For this review, take the finished solid that the model builds, in its own axes (mm). Face numbers are marked on the shaded views. A direction names the side the tool comes from. Coordinates: 2 decimals unless noted, no trailing zeros. Loops run counter-clockwise (first coordinate to the right, second up) from the corner with the lowest first, then second, coordinate; pieces in that order, holes last. Notation, with made-up numbers: M -15.75,38.5 L 18.25,38.5 A23 cw 18.25,58.5 Z; hole C 68.5,60.5 d11. An arc over 180 degrees is marked long. Use one line per item in the form item = value.
```python
from build123d import *

# Parameters (mm, degrees)
SKETCH1_R                      = 12.5
BOSS_EXTRUDE1_DEPTH            = 17.6
SKETCH2_R                      = 6.875
CUT_EXTRUDE1_DEPTH             = 50.8
SKETCH3_R                      = 8
CUT_EXTRUDE3_DEPTH             = 15.6
CUT_EXTRUDE4_DEPTH             = 18.6
BOSS_EXTRUDE2_DEPTH            = 17.6
FILLET1_R                      = 4
SKETCH6_W                      = 25
SKETCH6_H                      = 20.775
BOSS_EXTRUDE3_DEPTH            = 20
M4X0_7_TAPPED_HOLE2_AT_2_COUNT = 2
M4X0_7_TAPPED_HOLE2_AT_2_PITCH = 12.206555616
M4X0_7_TAPPED_HOLE1_D          = 3.3
M4X0_7_TAPPED_HOLE1_DEPTH      = 7
M4X0_7_TAPPED_HOLE1_TIP        = 0.991420021
FILLET4_R                      = 1
FILLET6_R                      = 1
FILLET7_R                      = 2
CUT_EXTRUDE6_DEPTH             = 15.6
FILLET8_R                      = 5
BOSS_EXTRUDE4_DEPTH            = 17.6
FILLET11_R                     = 1


with BuildPart() as part:
    # Sketch1 → Boss-Extrude1 (new body)
    with BuildSketch(Plane(origin=(0, 0, 0), x_dir=(1, 0, 0), z_dir=(0, 1, 0))):
        Circle(SKETCH1_R)
    extrude(amount=BOSS_EXTRUDE1_DEPTH)

    # Sketch2 → Cut-Extrude1 (cut)
    with BuildSketch(Plane(origin=(0, 17.6, 0), x_dir=(1, 0, 0), z_dir=(0, 1, 0))):
        Circle(SKETCH2_R)
    extrude(amount=-CUT_EXTRUDE1_DEPTH, mode=Mode.SUBTRACT)

    # Sketch3 → Cut-Extrude3 (cut)
    with BuildSketch(Plane(origin=(0, 17.6, 0), x_dir=(1, 0, 0), z_dir=(0, 1, 0))):
        Circle(SKETCH3_R)
    extrude(amount=-CUT_EXTRUDE3_DEPTH, mode=Mode.SUBTRACT)

    # Sketch4 → Cut-Extrude4 (cut, through all)
    with BuildSketch(Plane(origin=(0, 17.6, 0), x_dir=(1, 0, 0), z_dir=(0, 1, 0))):
        with BuildLine():
            ThreePointArc((-2.736161147, 7.517540966), (2.405646396, 7.629735606), (6.553216354, 4.588611491))
            Line((6.553216354, 4.588611491), (10.239400554, 7.169705454))
            ThreePointArc((10.239400554, 7.169705454), (3.758822494, 11.921461884), (-4.275251792, 11.74615776))
            Line((-4.275251792, 11.74615776), (-2.736161147, 7.517540966))
        make_face()
    extrude(amount=-CUT_EXTRUDE4_DEPTH, mode=Mode.SUBTRACT)

    # Sketch5 → Boss-Extrude2 (add, through all)
    with BuildSketch(Plane(origin=(0, 17.6, 0), x_dir=(1, 0, 0), z_dir=(0, 1, 0))):
        with BuildLine():
            Line((8.100371818, -9.520187835), (32.472052675, 11.216764019))
            Line((32.472052675, 11.216764019), (23.399636239, 21.879374394))
            Line((23.399636239, 21.879374394), (10.717665156, 11.088759446))
            Line((10.717665156, 11.088759446), (10.239400554, 7.169705454))
            ThreePointArc((10.239400554, 7.169705454), (12.398586499, -1.589041484), (8.100371818, -9.520187835))
        make_face()
    extrude(amount=-BOSS_EXTRUDE2_DEPTH)

    # Fillet1
    fillet1_edges = [part.edges().sort_by_distance(p)[0] for p in [
        (-2.736161147, 9.8, -7.517540966),
    ]]
    fillet(fillet1_edges, radius=FILLET1_R)

    # Sketch6 → Boss-Extrude3 (add)
    with BuildSketch(Plane(origin=(24.371680857, 0, -20.736951854), x_dir=(-0.648029745, 0, -0.761615027), z_dir=(0.761615027, 0, -0.648029745))):
        with Locations((0, 10.3875)):
            Rectangle(SKETCH6_W, SKETCH6_H)
    extrude(amount=BOSS_EXTRUDE3_DEPTH)

    # Sketch9 → M4x0.7 Tapped Hole2 (revolve, cut)
    with BuildSketch(Plane(origin=(25.410689361, 15.3875, -38.033496634), x_dir=(-0.761615027, 0, 0.648029745), z_dir=(0, 1, 0))):
        Polygon((0, 0), (0, 7.991420021), (1.65, 7), (1.65, 0), align=None)
    m4x0_7_tapped_hole2 = revolve(axis=Axis((21.295700477, 15.3875, -42.869752054), (0.648029745, 0, 0.761615027)), mode=Mode.SUBTRACT)

    # M4x0.7 Tapped Hole2 at 2: M4x0.7 Tapped Hole2 ×2
    with Locations(*[Vector(-0.436757539, -0.819231921, 0.371620657) * (i * M4X0_7_TAPPED_HOLE2_AT_2_PITCH) for i in range(1, M4X0_7_TAPPED_HOLE2_AT_2_COUNT)]):
        add(m4x0_7_tapped_hole2, mode=Mode.SUBTRACT)

    # Mirror1: M4x0.7 Tapped Hole2 across plane
    add(m4x0_7_tapped_hole2.mirror(Plane(origin=(0, 0, 0), x_dir=(-0.761615027, 0, 0.648029745), z_dir=(-0.648029745, 0, -0.761615027))), mode=Mode.SUBTRACT)

    # Mirror1 copy 1 sketch → Mirror1 copy 1 (revolve, cut)
    with BuildSketch(Plane(origin=(36.280127809, 5.3875, -14.456912746), x_dir=(-0.761615027, 0, 0.648029745), z_dir=(0, 1, 0))):
        Polygon((0, 0), (0, -7.991420021), (1.65, -7), (1.65, 0), align=None)
    revolve(axis=Axis((40.395116693, 5.3875, -9.620657326), (0.648029745, 0, 0.761615027)), mode=Mode.SUBTRACT)

    # M4x0.7 Tapped Hole1
    with Locations(Plane(origin=(0, 17.6, 0), x_dir=(1, 0, 0), z_dir=(0, 1, 0))):
        with Locations((20.785019884, 12.607162838), (15.760988598, 3.080405276)):
            Hole(M4X0_7_TAPPED_HOLE1_D / 2, depth=M4X0_7_TAPPED_HOLE1_DEPTH)
            with Locations((0, 0, -(M4X0_7_TAPPED_HOLE1_DEPTH + M4X0_7_TAPPED_HOLE1_TIP / 2))):  # 118° drill point
                Cone(0, M4X0_7_TAPPED_HOLE1_D / 2, M4X0_7_TAPPED_HOLE1_TIP, mode=Mode.SUBTRACT)

    # Fillet4
    fillet4_edges = [part.edges().sort_by_distance(p)[0] for p in [
        (27.935844457, 17.6, -16.548069207),
    ]]
    fillet(fillet4_edges, radius=FILLET4_R)

    # Fillet6
    fillet6_edges = [part.edges().sort_by_distance(p)[0] for p in [
        (-2.736161147, 1, -7.517540966),
        (6.553216354, 1, -4.588611491),
    ]]
    fillet(fillet6_edges, radius=FILLET6_R)

    # Fillet7
    fillet7_edges = [part.edges().sort_by_distance(p)[0] for p in [
        (23.399636239, 8.8, -21.879374394),
    ]]
    fillet(fillet7_edges, radius=FILLET7_R)

    # Sketch13 → Cut-Extrude6 (cut)
    with BuildSketch(Plane(origin=(0, 17.6, 0), x_dir=(1, 0, 0), z_dir=(0, 1, 0))):
        Polygon((7.237831979, 3.407900857), (11.336580589, 16.160351586), (5.142300877, 6.128355545), (6.34884573, 4.867459081), align=None)
    extrude(amount=-CUT_EXTRUDE6_DEPTH, mode=Mode.SUBTRACT)

    # Fillet8
    fillet8_edges = [part.edges().sort_by_distance(p)[0] for p in [
        (7.237831979, 9.8, -3.407900857),
    ]]
    fillet(fillet8_edges, radius=FILLET8_R)

    # Sketch14 → Boss-Extrude4 (add)
    with BuildSketch(Plane(origin=(0, 17.6, 0), x_dir=(1, 0, 0), z_dir=(0, 1, 0))):
        Polygon((7.926350274, 5.550090213), (9.325919645, 9.904575236), (10.717665156, 11.088759446), (10.239400554, 7.169705454), align=None)
    extrude(amount=-BOSS_EXTRUDE4_DEPTH)

    # Fillet11
    fillet11_edges = [part.edges().sort_by_distance(p)[0] for p in [
        (9.325919645, 8.8, -9.904575236),
    ]]
    fillet(fillet11_edges, radius=FILLET11_R)


solid = part.part
```
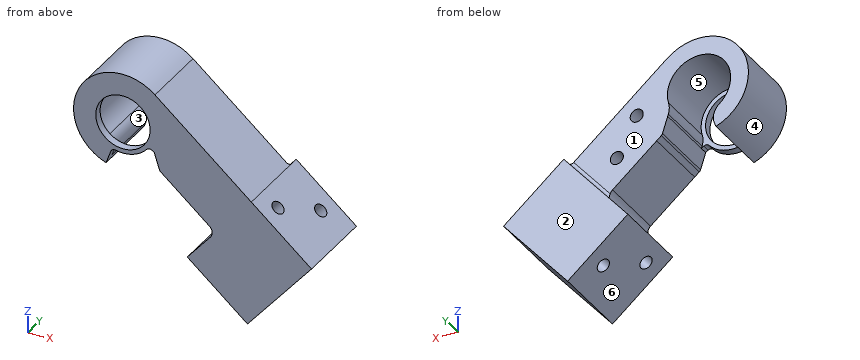
1. Consider section D-D on y = 19.75. Write out the cut boundary in (x, z).
Computed values:
outline = M 16.27,-30.26 L 31.5,-43.22 L 47.7,-24.18 L 32.47,-11.22 Z
2. Consider section B-B on y = 12.5. Write out the cut boundary in (x, z).
Computed values:
outline = M -5.09,-6.18 A8 cw long 7.7,-2.15 A5 ccw 7.76,-5.03 L 9.24,-9.63 A1 ccw 9.54,-10.09 L 21.88,-20.58 A2 cw 22.1,-23.4 L 16.27,-30.26 L 31.5,-43.22 L 47.7,-24.18 L 8.1,9.52 A12.5 ccw long -4.28,-11.75 L -3.87,-10.63 A4 ccw Z; hole C 15.76,-3.08 d3.3; hole C 20.79,-12.61 d3.3
3. Consider section C-C on z = 0. Write out the cut boundary in (x, y) (3 decimals), plus the area to 3 significant figures.
Computed values:
outline = M -12.5,0 L -6.875,0 L -6.875,2 L -8,2 L -8,17.6 L -12.5,17.6 Z; M 6.875,0 L 19.289,0 L 19.289,17.6 L 8,17.6 L 8,2 L 6.875,2 Z
area = 282 mm2
4. Draft analysis for pull direction Z (two halves, no side actions). For the marked faces 4, 5 and 6, state which applies: +Z half, -Z half, draft (parallel to the pull), parting line (faces both ways), or undercut.
Computed values:
face_4 = parting line
face_5 = undercut
face_6 = -Z half
5. Wall thickness on line 1 along Z through (x, y) = (0, 1.35) (3 decimals); line 2 along Y through (x, z) = (27, -36.5) (3 decimals); line 3 along Y through (x, z) = (29.5, -33) (3 decimals): over which ranges is each line inside the solid? List them lowest first. Write a range as from..to.
Computed values:
line_1 = -8..-6.875, 6.875..12.5
line_2 = 0..13.752, 17.023..20.775
line_3 = 0..13.744, 17.031..20.775
6. Consider section A-A on x = 0. Write out the cut boundary in (y, z) (3 decimals), plus the area to 3 significant figures.
Computed values:
outline = M 0,-8 L 2,-8 L 2,-6.875 L 0,-6.875 Z; M 0,6.875 L 2,6.875 L 2,8 L 17.6,8 L 17.6,12.5 L 0,12.5 Z
area = 83.7 mm2
7. For pin 1 Ø8 at (x, y) = (6.5, 7.5) entering from +Z; pin 2 Ø10 at (x, z) = (12.5, -4) entering from +Y; pin 3 Ø8 at (x, z) = (32, -3.5) entering from -Y; pin 4 Ø4 at (x, y) = (24, 11) entering from -Z, all flat-tipped, find the tip position at first contact; note any pin that passes through.
Computed values:
pin_1 = 12.25
pin_2 = 17.6
pin_3 = through
pin_4 = -38.53
8. Tool access review of the marked faces 1, 2 and 3: name each direction out of +Z, -Z, +X, -X, +Y, -Y from which nothing blocks a thin tool from reaching the whole face with its end or side.
Computed values:
face_1 = +Z, -X, +Y
face_2 = +Z, -Z, +X, -X, +Y
face_3 = +Y
